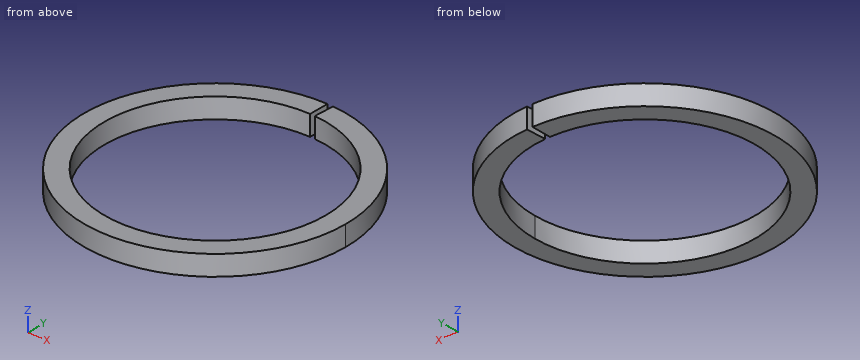
Autodesk Inventor part; units mm, degrees
ref_plane "YZ Plane" through (0, 0, 0) normal (1, 0, 0) x (0, 1, 0)
ref_plane "XZ Plane" through (0, 0, 0) normal (0, 1, 0) x (-1, 0, 0)
ref_plane "XY Plane" through (0, 0, 0) normal (0, 0, 1) x (1, 0, 0)
sketch "Sketch13" plane through (0, 0, 0) normal (0, 0, 1) x (1, 0, 0)
  circle A0 centre (0, 0) radius 33
  circle A1 centre (0, 0) radius 39.038
  line L0 (0, 0) -> (0, 39.038)
  line L1 (0, 0) -> (1.7028, 39.0008)
  line L2 (0, 0) -> (39.038, 0) construction
  point P0 (1.4394, 32.9686)
  point P1 (0, 33)
  dimension "d62" = 66
  dimension "d63" = 78.076
  dimension "d64" = 87.5
extrude "Extrusion12" add sketch "Sketch13" along normal blind 6 contours A0 L1 A1 L0 picked at (-2.8956, 36.6991)
sketch "Sketch4" plane through (40, -2.75, -25.3875) normal (1, 0, 0) x (0, 0, -1)
  line L0 (-51.025, 0.25) -> (-51.6313, 0.25)
  line L1 (-51.025, 0.25) -> (-55.267, 0.25)
  line L2 (-55.267, 0.25) -> (-55.267, 5.25)
  line L3 (-55.267, 5.25) -> (-51.025, 5.25)
  line L4 (-51.025, 5.25) -> (-51.025, 0.25)
  point P0 (-25.3875, 2.75)
  point P1 (-51.6313, 0.25)
  dimension "d33" = 4.242
  dimension "d34" = 5
sketch "Sketch5" plane through (40, -2.75, -25.3875) normal (1, 0, 0) x (0, 0, -1)
  line L0 (-51.6563, 0.25) -> (-55.267, 0.25)
  line L1 (-55.267, 5.25) -> (-51.6563, 5.25)
  line L2 (-55.267, 0.25) -> (-52.267, 0.25)
  line L3 (-52.267, 0.25) -> (-52.267, 5.25)
  line L4 (-52.267, 5.25) -> (-55.267, 5.25)
  line L5 (-55.267, 5.25) -> (-55.267, 0.25)
  point P0 (-25.3875, 2.75)
  point P1 (-55.267, 5.25)
  point P2 (-52.267, 0.25)
  dimension "d37" = 3
sketch "Sketch6" plane through (220, -2.75, -25.3875) normal (1, 0, 0) x (0, 0, -1)
  line L0 (-51.6563, 0.25) -> (-55.267, 0.25)
  line L1 (-55.267, 0.25) -> (-51.025, 0.25)
  line L2 (-51.025, 0.25) -> (-51.025, 5.25)
  line L3 (-51.025, 5.25) -> (-55.267, 5.25)
  line L4 (-55.267, 5.25) -> (-55.267, 0.25)
  point P0 (-25.3875, 2.75)
  dimension "d40" = 4.242
sketch "Sketch7" plane through (30, -2.75, -25.3875) normal (-1, 0, 0) x (0, 0, 1)
  line L0 (55.267, 0.25) -> (55.267, 5.25)
  line L1 (55.267, 0.25) -> (58.267, 0.25)
  line L2 (58.267, 0.25) -> (58.267, 5.25)
  line L3 (58.267, 5.25) -> (55.267, 5.25)
  line L4 (55.267, 5.25) -> (55.267, 0.25)
  point P0 (25.3875, 2.75)
  dimension "d43" = 3
  dimension "d44" = 5
sketch "Sketch8" plane through (30, -2.75, -25.3875) normal (-1, 0, 0) x (0, 0, 1)
  line L0 (51.6563, 0.25) -> (58.267, 0.25)
  line L1 (58.267, 5.25) -> (51.6563, 5.25)
  line L2 (58.267, 0.25) -> (57.025, 0.25)
  line L3 (57.025, 0.25) -> (57.025, 5.25)
  line L4 (57.025, 5.25) -> (58.267, 5.25)
  line L5 (58.267, 5.25) -> (58.267, 0.25)
  point P0 (25.3875, 2.75)
  point P1 (57.025, 0.25)
  dimension "d47" = 1.242
sketch "Sketch9" plane through (40, -2.75, -25.3875) normal (1, 0, 0) x (0, 0, -1)
  line L0 (-52.267, 0.25) -> (-51.025, 0.25)
  line L1 (-51.025, 5.25) -> (-51.025, 0.25)
  line L2 (-52.267, 0.25) -> (-51.025, 0.25)
  line L3 (-51.025, 0.25) -> (-51.025, 5.25)
  line L4 (-51.025, 5.25) -> (-52.267, 5.25)
  line L5 (-52.267, 5.25) -> (-52.267, 0.25)
  point P0 (-25.3875, 2.75)
properties part number "4002_Bias_Coil_Holder_Tube_Mount_Layer2_MPSv2_v1" material "Acetal Resin, White"
Geometry check sheet. Reference: the model listing, model coordinates, mm. Round coordinates to 2 decimals unless told otherwise and drop trailing zeros. Write each loop counter-clockwise with the first axis right and the second up, starting at its lowest first coordinate (ties: lowest second). Pieces come first, ordered by that corner, then holes.
Item 1: Material ranges on line 1 along X through (y, z) = (0, 2.5); line 2 along Y through (x, z) = (29.5, 2.25); line 3 along Y through (x, z) = (20, 1.5), recorded low to high.
Determined:
line 1: x = -39.04 to -33, 33 to 39.04
line 2: y = -25.57 to -14.79, 14.79 to 25.57
line 3: y = -33.53 to -26.25, 26.25 to 33.53
Item 2: Section check A-A (x = 16). Record the boundary of the cut face in (y, z).
Determined:
outline: (-35.61, 0) - (-28.86, 0) - (-28.86, 6) - (-35.61, 6) - close; (28.86, 0) - (35.61, 0) - (35.61, 6) - (28.86, 6) - close
Item 3: Section check C-C (z = 4.4). Record the boundary of the cut face in (x, y).
Determined:
outline: (0, 33) - (0, 39.04) arc R39.04 ccw (long way) to (1.7, 39) - (1.44, 32.97) arc R33 cw (long way) to start
Item 4: Go/stop test with flat-tipped pins: pin 1 Ø2 at (x, z) = (-5, 2) entering from +Y; pin 2 Ø2 at (x, y) = (26, -17) entering from +Z; pin 3 Ø2 at (y, z) = (-16.5, 4.5) entering from +X; pin 4 Ø2 at (x, z) = (-6.5, 2) entering from +Y. Record where each tip stops, or that it passes through.
Determined:
pin 1: stops at y = 38.83
pin 2: passes through
pin 3: stops at x = 35.83
pin 4: stops at y = 38.65
Item 5: Section check B-B (y = 9.5). Record the boundary of the cut face in (x, z).
Determined:
outline: (-37.86, 0) - (-31.6, 0) - (-31.6, 6) - (-37.86, 6) - close; (31.6, 0) - (37.86, 0) - (37.86, 6) - (31.6, 6) - close
